from build123d import *
from build123d.topology import SkipClean

# Parameters (mm, degrees)
BOSS_EXTRUDE1_DEPTH = 203.2
CUT_EXTRUDE1_DEPTH  = 204.2
BOSS_EXTRUDE2_DEPTH = 203.2
FILLET1_R           = 0.508
BOSS_EXTRUDE3_DEPTH = 203.2
CUT_EXTRUDE2_DEPTH  = 204.2
FILLET2_R           = 0.381


with BuildPart() as part:
    # Sketch1 → Boss-Extrude1 (new body)
    with BuildSketch(Plane(origin=(0, 0, 0), x_dir=(1, 0, 0), z_dir=(0, 1, 0))):
        with BuildLine():
            Line((101.58476, 5.338063609), (101.58476, 6.354063609))
            ThreePointArc((101.58476, 6.354063609), (50.79238, 19.05), (0, 6.354063609))
            Line((0, 6.354063609), (0, 5.338063609))
            Line((0, 5.338063609), (1.338554634, 5.338063609))
            ThreePointArc((1.338554634, 5.338063609), (45.188812602, 17.378377427), (90.062082389, 10.016044959))
            ThreePointArc((90.062082389, 10.016044959), (91.218156641, 9.549225792), (92.368682931, 9.068895628))
            ThreePointArc((92.368682931, 9.068895628), (96.251044015, 7.328911154), (100.06076, 5.435148318))
            Line((100.06076, 5.435148318), (100.06076, 4.322063609))
            ThreePointArc((100.06076, 4.322063609), (100.209549755, 3.962853364), (100.56876, 3.814063609))
            Line((100.56876, 3.814063609), (100.82276, 3.814063609))
            Line((100.82276, 3.814063609), (101.58476, 5.338063609))
        make_face()
    extrude(amount=BOSS_EXTRUDE1_DEPTH)

    # Sketch3 → Cut-Extrude1 (cut, through all)
    with BuildSketch(Plane(origin=(0, 203.2, 0), x_dir=(1, 0, 0), z_dir=(0, 1, 0))):
        Polygon((100.06076, 2.923708758), (101.58476, 2.923708758), (101.58476, 5.592063609), (100.06076, 5.435148318), align=None)
        Polygon((0, 5.592063609), (0.4067845, 4.474432381), (0, 4.474432381), align=None)
    extrude(amount=-CUT_EXTRUDE1_DEPTH, mode=Mode.SUBTRACT)

    # Sketch2 → Boss-Extrude2 (add)
    with BuildSketch(Plane(origin=(0, 203.2, 0), x_dir=(1, 0, 0), z_dir=(0, 1, 0))):
        with BuildLine():
            Line((98.79076, 4.639563606), (101.238078351, 4.639563606))
            Line((101.238078351, 4.639563606), (101.58476, 5.592063609))
            Line((101.58476, 5.592063609), (100.06076, 5.435148318))
            ThreePointArc((100.06076, 5.435148318), (99.355551952, 5.800115132), (98.647640508, 6.159810213))
            ThreePointArc((98.647640508, 6.159810213), (96.114471858, 2.891665388), (99.718733273, 0.865088556))
            ThreePointArc((99.718733273, 0.865088556), (99.858345852, 0.953692868), (99.947271519, 1.093100982))
            Line((99.947271519, 1.093100982), (100.173716674, 1.715253931))
            ThreePointArc((100.173716674, 1.715253931), (100.127790714, 2.064096228), (99.815693785, 2.226563606))
            Line((99.815693785, 2.226563606), (98.79076, 2.226563606))
            ThreePointArc((98.79076, 2.226563606), (97.58426, 3.433063606), (98.79076, 4.639563606))
        make_face()
        with BuildLine():
            ThreePointArc((1.769066215, 2.226563606), (1.456969286, 2.064096228), (1.411043326, 1.715253931))
            Line((1.411043326, 1.715253931), (1.637488481, 1.093100982))
            ThreePointArc((1.637488481, 1.093100982), (1.726414148, 0.953692868), (1.866026727, 0.865088556))
            ThreePointArc((1.866026727, 0.865088556), (5.470288142, 2.891665388), (2.937119492, 6.159810213))
            ThreePointArc((2.937119492, 6.159810213), (2.136102242, 5.752311703), (1.338554634, 5.338063609))
            Line((1.338554634, 5.338063609), (0.09244844, 5.338063609))
            Line((0.09244844, 5.338063609), (0.346681649, 4.639563606))
            Line((0.346681649, 4.639563606), (2.794, 4.639563606))
            ThreePointArc((2.794, 4.639563606), (4.0005, 3.433063606), (2.794, 2.226563606))
            Line((2.794, 2.226563606), (1.769066215, 2.226563606))
        make_face()
    extrude(amount=-BOSS_EXTRUDE2_DEPTH)

    # Fillet1
    fillet1_edges = [part.edges().sort_by_distance(p)[0] for p in [
        (101.238078351, 101.6, -4.639563606),
        (0.346681649, 101.6, -4.639563606),
    ]]
    fillet(fillet1_edges, radius=FILLET1_R)

    # Sketch4 → Boss-Extrude3 (add, through all)
    with BuildSketch(Plane(origin=(0, 203.2, 0), x_dir=(1, 0, 0), z_dir=(0, 1, 0))):
        with BuildLine():
            ThreePointArc((3.991870192, 5.886782672), (5.288114571, 4.544379384), (5.419434578, 2.682914602))
            ThreePointArc((5.419434578, 2.682914602), (50.79238, -7.212984057), (96.165325422, 2.682914602))
            ThreePointArc((96.165325422, 2.682914602), (96.296645429, 4.544379384), (97.592889808, 5.886782672))
            ThreePointArc((97.592889808, 5.886782672), (50.79238, -4.926984057), (3.991870192, 5.886782672))
        make_face()
        with BuildLine():
            ThreePointArc((2.937119492, 6.159810213), (3.478250935, 6.076438514), (3.991870192, 5.886782672))
            ThreePointArc((3.991870192, 5.886782672), (3.588373028, 6.084817853), (3.185713825, 6.284551329))
            ThreePointArc((3.185713825, 6.284551329), (3.061375909, 6.222261981), (2.937119492, 6.159810213))
        make_face()
        with BuildLine():
            ThreePointArc((98.399046175, 6.284551329), (97.996386972, 6.084817853), (97.592889808, 5.886782672))
            ThreePointArc((97.592889808, 5.886782672), (98.106509065, 6.076438514), (98.647640508, 6.159810213))
            ThreePointArc((98.647640508, 6.159810213), (98.523384091, 6.222261981), (98.399046175, 6.284551329))
        make_face()
    extrude(amount=-BOSS_EXTRUDE3_DEPTH)

    # Sketch5 → Cut-Extrude2 (cut, through all)
    with SkipClean():  # keep this step's faces unmerged: merging them makes the solid invalid here
        with BuildSketch(Plane(origin=(0, 203.2, 0), x_dir=(1, 0, 0), z_dir=(0, 1, 0))):
            with BuildLine():
                ThreePointArc((98.399046175, 6.284551329), (98.468630342, 6.31928211), (98.538189172, 6.354063609))
                Line((98.538189172, 6.354063609), (101.58476, 6.354063609))
                ThreePointArc((101.58476, 6.354063609), (50.79238, 19.05), (0, 6.354063609))
                Line((0, 6.354063609), (3.046570828, 6.354063609))
                ThreePointArc((3.046570828, 6.354063609), (3.116129658, 6.31928211), (3.185713825, 6.284551329))
                ThreePointArc((3.185713825, 6.284551329), (50.79238, 17.526), (98.399046175, 6.284551329))
            make_face()
        extrude(amount=-CUT_EXTRUDE2_DEPTH, mode=Mode.SUBTRACT)

    # Fillet2
    fillet2_edges = [part.edges().sort_by_distance(p)[0] for p in [
        (5.419434578, 101.6, -2.682914602),
        (96.165325422, 101.6, -2.682914602),
    ]]
    fillet(fillet2_edges, radius=FILLET2_R)


solid = part.part
Read the model definition and answer for the solid it produces. Units are mm, in the model's axes. Give positions to 0.01 mm unless a question says otherwise; leave off trailing zeros. Write each loop counter-clockwise with the first axis right and the second up, starting at its lowest first coordinate (ties: lowest second). Pieces come first, ordered by that corner, then holes. Notation, with made-up numbers: (62, 10) - (119, 10) arc R38 cw to (119, 49) - close; hole circle Ø3 at (58.5, 50). An arc over 180 degrees is marked (long way). Use CSV: the item, a comma, the result in double quotes. Start each with the question number.
(1) Given P1, Ø1.7, axis at x = 100, y = 68, coming from the +Z side; P2, Ø6, axis at x = 43, y = 49.5, coming from the -Z side; P3, Ø12, axis at x = 73.5, y = 91.5, coming from the +Z side, each flat-ended and moving along its own axis, determine where each tip first touches the part or whether it passes through.
(2) Find section A-A (z = 2.25). Give the vertices of the cut face in (x, y), plus the area to 3 significant figures.
(3) Find section B-B (x = 85.5). Give the vertices of the cut face in (y, z), plus the area to 3 significant figures.
(4) Determine the mould class of faces 1 (the cylindrical face through (97.7, 103.02, -0.93)), 2 (the cylindrical face through (51.471, 103.022, 4.925)), 3 (the flat face through (50.6, 203.2, 5.4)) for opening direction X: +X half, -X half, draft (parallel to the pull), parting line (faces both ways), or undercut.
(5) Consider line 1 along X through (y, z) = (132, -2.5); line 2 along X through (y, z) = (73.5, -5.25); line 3 along Z through (x, y) = (26.5, 172.5). Determine where each line is inside the solid, lowest interval first.
Findings below:
1,P1,"z = -0.73"
1,P2,"z = 4.38"
1,P3,"z = 5.92"
2,outline,"(18.28, 0) - (27.04, 0) - (27.04, 203.2) - (18.28, 203.2) - close; (74.54, 0) - (83.3, 0) - (83.3, 203.2) - (74.54, 203.2) - close"
2,area,"3,560 mm2"
3,outline,"(0, -0.88) - (203.2, -0.88) - (203.2, 1.54) - (0, 1.54) - close"
3,area,"491 mm2"
4,face 1,"undercut"
4,face 2,"undercut"
4,face 3,"draft"
5,line 1,"3.56 to 5.45, 5.82 to 11.68, 89.9 to 95.76, 96.13 to 98.03"
5,line 2,"0.12 to 5.32, 96.27 to 101.46"
5,line 3,"2.12 to 4.47"
